from build123d import *

# Parameters (mm, degrees)
SKETCH1_W           = 23.622
SKETCH1_H           = 20.1676
BOSS_EXTRUDE1_DEPTH = 5.715
SKETCH4_W           = 11.43
SKETCH4_H           = 1.9939
BOSS_EXTRUDE4_DEPTH = 4.4958
BOSS_EXTRUDE5_START = -0.9779
SKETCH5_R           = 5.715
BOSS_EXTRUDE5_DEPTH = 5.969
SKETCH6_R           = 2.54
BOSS_EXTRUDE6_DEPTH = 3.1242
SKETCH7_R           = 1.016
CUT_EXTRUDE1_DEPTH  = 26.822810407
SKETCH8_W           = 6.0452
SKETCH8_H           = 3.302
BOSS_EXTRUDE7_DEPTH = 1.4097
BOSS_EXTRUDE8_DEPTH = 4.572


with BuildPart() as part:
    # Sketch1 → Boss-Extrude1 (new, symmetric)
    with BuildSketch(Plane.XY):
        with Locations((0, 10.0838)):
            Rectangle(SKETCH1_W, SKETCH1_H)
    extrude(amount=BOSS_EXTRUDE1_DEPTH, both=True)

    # Sketch4 → Boss-Extrude4 (add)
    with BuildSketch(Plane.ZY.offset(11.811)):
        with Locations((0, 18.19275)):
            Rectangle(SKETCH4_W, SKETCH4_H)
    boss_extrude4 = extrude(amount=BOSS_EXTRUDE4_DEPTH)

    # Mirror1: Boss-Extrude4 across plane
    add(boss_extrude4.mirror(Plane(origin=(0, 0, 0), x_dir=(0, 0, 1), z_dir=(1, 0, 0))))

    # Sketch5 → Boss-Extrude5 (add)
    with BuildSketch(Plane(origin=(0, 20.1676, 0), x_dir=(1, 0, 0), z_dir=(0, 1, 0)).offset(BOSS_EXTRUDE5_START)):
        with Locations((-5.7912, 0)):
            Circle(SKETCH5_R)
    extrude(amount=BOSS_EXTRUDE5_DEPTH)

    # Sketch6 → Boss-Extrude6 (add)
    with BuildSketch(Plane(origin=(0, 25.1587, 0), x_dir=(1, 0, 0), z_dir=(0, 1, 0))):
        with Locations(Location((-5.7912, 0, 0), (0, 0, 180))):
            Circle(SKETCH6_R)
    extrude(amount=BOSS_EXTRUDE6_DEPTH)

    # Sketch7 → Cut-Extrude1 (cut, through all)
    with BuildSketch(Plane(origin=(0, 19.1897, 0), x_dir=(1, 0, 0), z_dir=(0, 1, 0))):
        with Locations(Location((-13.6525, 3.302, 0), (0, 0, 180))):
            Circle(SKETCH7_R)
        with Locations(Location((-13.6525, -3.302, 0), (0, 0, 180))):
            Circle(SKETCH7_R)
        with Locations(Location((-14.1605, 0, 0), (0, 0, 180))):
            Circle(SKETCH7_R)
    cut_extrude1 = extrude(amount=-CUT_EXTRUDE1_DEPTH, mode=Mode.SUBTRACT)

    # Mirror2: Cut-Extrude1 across plane
    add(cut_extrude1.mirror(Plane(origin=(0, 0, 0), x_dir=(0, 0, 1), z_dir=(1, 0, 0))), mode=Mode.SUBTRACT)

    # Sketch8 → Boss-Extrude7 (add)
    with BuildSketch(Plane.ZY.offset(11.811)):
        with Locations((0, 3.175)):
            Rectangle(SKETCH8_W, SKETCH8_H)
    extrude(amount=BOSS_EXTRUDE7_DEPTH)

    # Sketch9 → Boss-Extrude8 (add)
    with BuildSketch(Plane.ZY.offset(13.2207)):
        with BuildLine():
            Line((1.651, 2.6924), (-1.651, 2.6924))
            ThreePointArc((-1.651, 2.6924), (-2.1336, 3.175), (-1.651, 3.6576))
            Line((-1.651, 3.6576), (1.651, 3.6576))
            ThreePointArc((1.651, 3.6576), (2.1336, 3.175), (1.651, 2.6924))
        make_face()
    extrude(amount=BOSS_EXTRUDE8_DEPTH)


solid = part.part
The model under review builds one solid part; all positions refer to its coordinate system, in mm. A direction names the side the tool comes from. Give positions to 0.01 mm unless a question says otherwise; leave off trailing zeros. Loops run counter-clockwise (first coordinate to the right, second up) from the corner with the lowest first, then second, coordinate; pieces in that order, holes last. Notation, with made-up numbers: (-9, 88) -> (17, 88) arc R28 ccw to (17, 111) -> close; hole circle Ø8 at (26.25, 73.5). An arc over 180 degrees is marked (long way). Answer as a JSON object with one key per item and string values. Group by question number.
Q1. Take a section at C-C (z = 0). State how many separate pieces and enclosed holes the cut face has, plus the area to 3 significant figures.
Q2. Draft analysis for pull direction Y (two halves, no side actions). For faces 1 (the flat face through (-13.221, 4, 0)), 2 (the flat face through (-11.811, 20, 0)), 3 (the flat face through (-13, 1.524, 0)), state which applies: pulls with the +Y half, pulls with the -Y half, needs draft (parallel to the pull), parting line crosses it, or undercut.
Q3. Tool access review of faces 4 (the flat face through (-15, 3.658, 0)), 5 (the flat face through (11.811, 20, 0)), 6 (the cylindrical face through (-15.475, 3.186, 2.133)), 7 (the flat face through (-13, 3, -3.023)): name each direction out of +Z, -Z, +X, -X, +Y, -Y from which nothing blocks a thin tool from reaching the whole face with its end or side.
Q4. Take a section at D-D (y = 24.25). Write out the cut boundary in (x, z) (3 decimals), plus the area to 3 significant figures.
Q5. Take a section at B-B (y = 16). Write out the cut boundary in (x, z) (3 decimals).
Q6. Take a section at A-A (x = -1.5). Write out the cut boundary in (y, z) (1 decimal).
Q7. Insertion check: pin 1 (8 mm diameter, centred on x = -8, y = 20.5, fed in from +Z) (3 decimals); pin 2 (5 mm diameter, centred on x = -15, z = 2, fed in from +Y); pin 3 (4 mm diameter, centred on y = 5.5, z = 3.5, fed in from -X); pin 4 (4 mm diameter, centred on x = -13.5, z = -1, fed in from +Y). Each pin has a flat end and moves straight along its axis. Give the tip position at first contact, or say it passes through.
Q8. Wall thickness on line 1 along Y through (x, z) = (-15.5, -0.75); line 2 along Y through (x, z) = (11.5, -0.25); line 3 along X through (y, z) = (14.5, -4): over which ranges is each line inside the solid? List them lowest first.
Answer below:
{
 "1": {"separate pieces": "3", "enclosed holes": "0", "area": "568 mm2"},
 "2": {"face 1": "undercut", "face 2": "needs draft", "face 3": "pulls with the -Y half"},
 "3": {"face 4": "+Z, -Z, -X", "face 5": "+Z, -Z, +X, +Y", "face 6": "+Z, -X", "face 7": "-Z, -X, -Y"},
 "4": {"outline": "circle Ø11.43 at (-5.791, 0)", "area": "103 mm2"},
 "5": {"outline": "(-11.811, -5.715) -> (11.811, -5.715) -> (11.811, 5.715) -> (-11.811, 5.715) -> close"},
 "6": {"outline": "(0, -5.7) -> (20.2, -5.7) -> (20.2, -3.8) -> (25.2, -3.8) -> (25.2, 3.8) -> (20.2, 3.8) -> (20.2, 5.7) -> (0, 5.7) -> close"},
 "7": {"pin 1": "stops at z = 5.715", "pin 2": "stops at y = 19.19", "pin 3": "stops at x = -13.22", "pin 4": "stops at y = 20.17"},
 "8": {"line 1": "y = 2.69 to 3.66, 17.2 to 19.19", "line 2": "y = 0 to 20.17", "line 3": "x = -11.81 to 11.81"}
}
